Can you work these out from the model? Positions are in its coordinate system, mm. Face numbers are marked on the shaded views. A direction names the side the tool comes from. Give positions to 0.01 mm unless a question says otherwise; leave off trailing zeros. Order: outer loops, then holes, each group sorted by start corner. A loop starts at its lowest first (then second) coordinate and runs counter-clockwise, first axis right, second up. Notation, with made-up numbers: (88.25, 89) - (122.25, 89) arc R21 ccw to (122.25, 124) - close; hole circle Ø10 at (-38.5, 56.25). An arc over 180 degrees is marked (long way). Write each question's results on one line, items separated by ' | '. Start each with the question number.
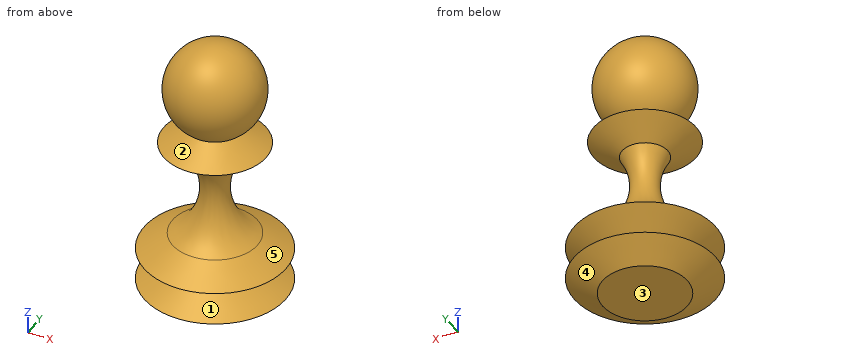
from build123d import *


with BuildPart() as f1:
    # F0 (on Front) → F1 (revolve)
    with BuildSketch(Plane.XZ):
        with BuildLine():
            Line((0, 57.020247), (0, 0))
            Line((0, 0), (9, 0))
            Line((9, 0), (15, 3.5))
            Line((15, 3.5), (9, 7))
            Line((9, 7), (15, 10.5))
            Line((15, 10.5), (9, 14))
            ThreePointArc((9, 14), (3.236656, 21.745631), (4.835254, 31.266944))
            Line((4.835254, 31.266944), (10.835254, 34.766944))
            Line((10.835254, 34.766944), (4.835254, 38.266944))
            ThreePointArc((4.835254, 38.266944), (9.683311, 49.516942), (0, 57.020247))
        make_face()
    revolve(axis=Axis((0, 0, 28.510124), (0, 0, -1)))


solid = f1.part
Q1. If we section it at C-C (z = 37): Please give me the cut outline in (x, y), plus the area to 3 significant figures.
Q2. If we section it at B-B (x = 0): Please give me the cut outline in (y, z).
Q3. Thinking about a two-plate mould opening in Z: for the marked faces 1, 2 and 3, which applies, released by +Z, released by -Z, zero draft, split by the parting line, or undercut?
Q4. Will these pins go through, and if not, where does the flat tip stop? P1, Ø2, axis at x = 7, y = 11, coming from the +Z side; P2, Ø8, axis at x = -5, y = -4.5, coming from the +Z side; P3, Ø2, axis at y = -2.5, z = 44, coming from the +X side.
Q5. If I drill on probe 1 along Z at (x, y) = (7, -2); probe 2 along Z at (x, y) = (-6.5, 10.75); probe 3 along Z at (x, y) = (10.25, -2), over which ranges is the centre line in solid material (lowest first)? Write a range as from..to.
Q6. If we section it at A-A (y = 7.5): State how many separate pieces and enclosed holes the cut face has, plus the area to 3 significant figures.
Q7. Which directions (+Z, -Z, +X, -X, +Y, -Y) give clear straight access to the entire face, cutting with the end or side of a thin tool? Please do the marked faces 4 and 5.
Findings below:
1) outline: circle Ø14.01 at (0, 0) | area: 154 mm2
2) outline: (-15, 3.5) - (-9, 0) - (9, 0) - (15, 3.5) - (9, 7) - (15, 10.5) - (9, 14) arc R12.31 cw to (4.84, 31.27) - (10.84, 34.77) - (4.84, 38.27) arc R10 ccw (long way) to (-4.84, 38.27) - (-10.84, 34.77) - (-4.84, 31.27) arc R12.31 cw to (-9, 14) - (-15, 10.5) - (-9, 7) - close
3) face 1: undercut | face 2: undercut | face 3: released by -Z
4) P1: stops at z = 12.23 | P2: stops at z = 56.64 | P3: stops at x = 9.56
5) probe 1: z = 0..15.21, 32.69..36.84, 40.16..53.88 | probe 2: z = 2.08..4.92, 9.08..11.92 | probe 3: z = 0.84..6.16, 7.84..13.16, 34.54..35
6) separate pieces: 3 | enclosed holes: 0 | area: 442 mm2
7) face 4: -Z | face 5: none
